Can you work these out from the model? Positions are in its coordinate system, mm. A direction names the side the tool comes from. Give positions to 0.01 mm unless a question says otherwise; leave off trailing zeros. Write each loop counter-clockwise with the first axis right and the second up, starting at its lowest first coordinate (ties: lowest second). Pieces come first, ordered by that corner, then holes.
Autodesk Inventor part; units mm, degrees
ref_plane "Work Plane1" through (0, 0, -15) normal (0, 0, 1) x (1, 0, 0)
ref_plane "YZ Plane" through (0, 0, 0) normal (1, 0, 0) x (0, 1, 0)
ref_plane "XZ Plane" through (0, 0, 0) normal (0, 1, 0) x (-1, 0, 0)
sketch "Sketch1" plane through (0, 0, 0) normal (0, 0, 1) x (1, 0, 0)
  line L0 (0, 0) -> (25, 0)
  line L1 (25, 0) -> (25, 40)
  line L2 (25, 40) -> (0, 40)
  line L3 (0, 40) -> (0, 0)
  dimension "d1" = 25
  dimension "d2" = 40
  dimension "d3" = 25
extrude "Extrusion1" add sketch "Sketch1" against normal blind 30
sketch "Sketch2" plane through (25, 0, 0) normal (1, 0, 0) x (0, 0, -1)
  line L0 (0, 0) -> (30, 0)
  circle A0 centre (15, 6.56) radius 2.46
extrude "Extrusion2" cut sketch "Sketch2" against normal blind 30
sketch "Sketch3" plane through (0, 0, 0) normal (-1, 0, 0) x (0, 0, 1)
  line L0 (0, 0) -> (-30, 0)
  line L1 (-25.05, 0) -> (-4.95, 0)
  line L2 (-4.95, 0) -> (-4.95, 33.12)
  line L3 (-4.95, 33.12) -> (-25.05, 33.12)
  line L4 (-25.05, 33.12) -> (-25.05, 0)
  dimension "d11" = 20.1
extrude "Extrusion3" cut sketch "Sketch3" against normal blind 20
sketch "Sketch4" plane through (0, 0, 0) normal (0, -1, 0) x (1, 0, 0)
  line L0 (20, -4.95) -> (20, -25.05)
  line L1 (20, -15) -> (25, -15)
  line L2 (25, 0) -> (25, -30)
  line L3 (20, -8.025) -> (25, -8.025)
  line L4 (25, -8.025) -> (25, -21.975)
  line L5 (25, -21.975) -> (20, -21.975)
  line L6 (20, -21.975) -> (20, -8.025)
  line L7 (20, -8.025) -> (25, -21.975) construction
  line L8 (25, -8.025) -> (20, -21.975) construction
  line L9 (25, -12.54) -> (25, -17.46)
  point P0 (0, 0)
  point P1 (22.5, -15)
  dimension "d14" = 13.95
extrude "Extrusion4" add sketch "Sketch4" along normal blind 15
sketch "Sketch5" plane through (20, 0, 0) normal (-1, 0, 0) x (0, 0, 1)
  circle A0 centre (-15, 6.56) radius 2.46
  circle A1 centre (-15, 6.56) radius 4.7025
  circle A2 centre (-15, 6.56) radius 2.46
  circle A3 centre (-15, 6.56) radius 2.46
  point P0 (0, 0)
  dimension "d17" = 9.405
extrude "Extrusion5" cut sketch "Sketch5" against normal blind 2.1
sketch "Sketch6" plane through (25, 0, 0) normal (1, 0, 0) x (0, 0, -1)
  circle A0 centre (15, 6.56) radius 4.7025
  line L0 (15, 6.56) -> (15, 23.56)
  circle A1 centre (15, 23.56) radius 2.46
  point P0 (0, 0)
  dimension "d20" = 17
  dimension "d21" = 4.92
extrude "Extrusion6" cut sketch "Sketch6" against normal blind 10 contours A1
sketch "Sketch7" plane through (20, 0, 0) normal (-1, 0, 0) x (0, 0, 1)
  circle A0 centre (-15, 23.56) radius 2.46
  circle A1 centre (-15, 23.56) radius 4.7025
  point P0 (0, 0)
  dimension "d24" = 9.405
extrude "Extrusion7" cut sketch "Sketch7" against normal blind 2.1
sketch "Sketch9" plane through (25, 0, 0) normal (1, 0, 0) x (0, 0, -1)
  circle A0 centre (15, 6.56) radius 2.46
  circle A1 centre (15, 6.56) radius 2.46
  circle A2 centre (15, 23.56) radius 2.46
  circle A3 centre (15, 23.56) radius 2.46
  line L0 (30, 40) -> (30, 0)
  line L1 (30, 0) -> (30, 40)
  line L2 (30, 40) -> (0, 40)
  line L3 (0, 40) -> (0, 0)
  line L4 (0, 0) -> (8.025, 0)
  line L5 (21.975, 0) -> (21.975, -15)
  line L6 (21.975, -15) -> (8.025, -15)
  line L7 (8.025, -15) -> (8.025, 0)
  line L8 (0, 0) -> (8.025, 0)
  line L9 (21.975, 0) -> (30, 0)
extrude "Extrusion8" add sketch "Sketch9" along normal blind 5
sketch "Sketch10" plane through (0, 40, 0) normal (0, 1, 0) x (1, 0, 0)
  line L0 (0, 30) -> (30, 30)
  line L1 (30, 0) -> (0, 0)
  line L2 (0, 30) -> (30, 30)
  line L3 (30, 30) -> (30, 0)
  line L4 (30, 0) -> (0, 0)
  line L5 (0, 0) -> (0, 30)
extrude "Extrusion9" add sketch "Sketch10" along normal blind 30
sketch "Sketch12" plane through (30, 0, 0) normal (1, 0, 0) x (0, 0, -1)
  circle A0 centre (15, 6.56) radius 2.46
  line L0 (15, 6.56) -> (15, 15.06)
  circle A1 centre (15, 15.06) radius 2.525
  point P0 (0, 0)
  dimension "d31" = 8.5
  dimension "d33" = 5.05
extrude "Extrusion10" cut sketch "Sketch12" against normal blind 30 contours A1
sketch "Sketch15" plane through (0, 0, -25.05) normal (-1, 0, 0) x (0, 0, 1)
  line L0 (0, 33.12) -> (20.1, 33.12)
  line L1 (20.1, 33.12) -> (20.1, 0)
  line L2 (0, 33.12) -> (20.1, 33.12)
  line L3 (20.1, 33.12) -> (20.1, 31.1)
  line L4 (20.1, 31.1) -> (0, 31.1)
  line L5 (0, 31.1) -> (0, 33.12)
  point P0 (25.05, 0)
  dimension "d57" = 2.02
extrude "Extrusion13" add sketch "Sketch15" against normal blind 20
sketch "Sketch17" plane through (0, 0, 0) normal (0, 0, 1) x (1, 0, 0)
  line L0 (0, 70) -> (30, 70)
  line L1 (30, 70) -> (50.0622, 90.0622)
  line L2 (30, 70) -> (80, 70) construction
  line L3 (11.9522, 97.2454) -> (0, 85.2932)
  line L4 (0, 70) -> (0, 85.2932)
  line L5 (0, 70) -> (0, 0)
  line L6 (0, 70) -> (30, 70)
  line L7 (10.923, 112.2849) -> (0, 120.567)
  line L8 (50.0622, 105.3553) -> (50.0622, 120.567)
  line L9 (50.0622, 105.3553) -> (50.0622, 90.0622)
  arc A0 (11.9522, 97.2454) -> (10.923, 112.2849) centre (4.8811, 104.3165) ccw
  line L10 (0, 144.567) -> (30, 144.567)
  line L11 (30, 144.567) -> (50.0622, 120.567)
  line L12 (4, 142.567) -> (0, 144.567)
  line L13 (4, 122.567) -> (0, 120.567)
  line L14 (4, 122.567) -> (8, 132.567)
  line L15 (8, 132.567) -> (4, 142.567)
  dimension "d61" = 45
  dimension "d62" = 32.0271
  dimension "d72" = 10
extrude "Extrusion14" add sketch "Sketch17" against normal blind 30
sketch "Sketch22" plane through (0, 0, 0) normal (0, 0, 1) x (1, 0, 0)
  line L0 (11.9522, 97.2454) -> (0, 85.2932)
  line L1 (0, 85.2932) -> (11.9522, 97.2454)
  arc A0 (11.9522, 97.2454) -> (10.923, 112.2849) centre (4.8811, 104.3165) ccw
  arc A1 (11.9522, 97.2454) -> (10.923, 112.2849) centre (4.8811, 104.3165) ccw
  line L2 (0, 120.567) -> (10.923, 112.2849)
  line L3 (10.923, 112.2849) -> (0, 120.567)
  line L4 (0, 120.567) -> (4, 122.567)
  line L5 (0, 120.567) -> (4, 122.567)
  line L6 (4, 122.567) -> (8, 132.567)
  line L7 (4, 122.567) -> (8, 132.567)
  line L8 (8, 132.567) -> (4, 142.567)
  line L9 (8, 132.567) -> (4, 142.567)
  line L10 (4, 142.567) -> (0, 144.567)
  line L11 (4, 142.567) -> (0, 144.567)
  line L12 (0, 144.567) -> (30, 144.567)
  line L13 (0, 144.567) -> (30, 144.567)
  line L14 (50.0622, 120.567) -> (30, 144.567)
  line L15 (30, 144.567) -> (50.0622, 120.567)
  line L16 (50.0622, 120.567) -> (50.0622, 90.0622)
  line L17 (50.0622, 120.567) -> (50.0622, 90.0622)
  line L18 (30, 70) -> (50.0622, 90.0622)
  line L19 (50.0622, 90.0622) -> (30, 70)
  line L20 (0, 0) -> (0, 85.2932)
  line L21 (0, 85.2932) -> (0, 55.2932)
  line L22 (0, 55.2932) -> (30, 55.2932)
  line L23 (30, 0) -> (30, 70)
  line L24 (30, 55.2932) -> (30, 70)
  dimension "d83" = 30
extrude "Extrusion15" add sketch "Sketch22" along normal blind 15
ref_plane "Work Plane1" through (0, 0, -15) normal (0, 0, 1) x (1, 0, 0)
mirror "Mirror1" about plane through (0, 0, -15) normal (0, 0, 1) of "Extrusion15"
properties part number "rec_c_20mm_x_60mm"
1) For pin 1 Ø16.5 at (x, z) = (10.5, 4) entering from -Y; pin 2 Ø2 at (x, z) = (37.5, -22.5) entering from +Y; pin 3 Ø22 at (x, y) = (6.5, 16.5) entering from +Z, each with a flat end and sliding along its axis, tell me the tip position at first contact or that it passes through.
Values follow:
pin 1: stops at y = 0
pin 2: stops at y = 136.79
pin 3: stops at z = 0
2) If we mould it in two halves opening along Y, with no side actions, what happens to faces 1 (the face through (15, 55.293, -37)), 2 (the face through (15, 28, 0)), 3 (the face through (22.1, 21.5, -13))? For each: +Y half, -Y half, draft (parallel to the pull), parting line (faces both ways), or undercut.
Values follow:
face 1: -Y half
face 2: draft
face 3: undercut
3) Suppose I cut it at B-B on z = -33.5. Write out the boundary of the cut face in (x, y), plus the area to 3 significant figures.
Values follow:
outline: (0, 55.29) - (30, 55.29) - (30, 70) - (50.06, 90.06) - (50.06, 120.57) - (30, 144.57) - (0, 144.57) - (4, 142.57) - (8, 132.57) - (4, 122.57) - (0, 120.57) - (10.92, 112.28) arc R10 cw to (11.95, 97.25) - (0, 85.29) - close
area: 3,280 mm2
4) For faces 4 (the face through (18, 0, -27)), 5 (the face through (30, 38, -15)), 6 (the face through (2.03, 121.58, -14.58)), 7 (the face through (22.1, 4.5, -13)), which set-ups out of +Z, -Z, +X, -X, +Y, -Y let a thin tool reach every point of the face, with its end or its side?
Values follow:
face 4: -Z, +X, -X, -Y
face 5: +Z, -Z, +X, -Y
face 6: +Z, -Z, -X
face 7: -X
5) Suppose I cut it at A-A on y = 15.06. Write out the boundary of the cut face in (x, z) (3 decimals), plus the area to 4 significant figures.
Values follow:
outline: (0, -30) - (30, -30) - (30, -17.525) - (20, -17.525) - (20, -25.05) - (0, -25.05) - close; (0, -4.95) - (20, -4.95) - (20, -12.475) - (30, -12.475) - (30, 0) - (0, 0) - close
area: 447.5 mm2
6) Suppose I cut it at D-D on y = 65. Write out the boundary of the cut face in (x, z).
Values follow:
outline: (0, -45) - (30, -45) - (30, 15) - (0, 15) - close
7) Suppose I cut it at C-C on z = -15. State how many separate pieces and enclosed holes the cut face has, plus the area to 3 significant figures.
Values follow:
separate pieces: 4
enclosed holes: 0
area: 4,300 mm2
8) Please list where these lines run through material, in increasing order: L1, parallel to Y at x = 20.75, z = -15 (1 decimal); L2, parallel to Y at x = 24, z = -15 (3 decimals); L3, parallel to Z at x = 24, y = 15.06 (3 decimals).
Values follow:
L1: y = -15 to 1.9, 11.3 to 12.5, 17.6 to 18.9, 28.3 to 144.6
L2: y = -15 to 4.1, 9.02 to 12.535, 17.585 to 21.1, 26.02 to 144.567
L3: z = -30 to -17.525, -12.475 to 0
